Geometry check sheet. Reference: drawing and pictorial views, mm from the part's lowest x, y, z. Give positions to 0.01 mm unless a question says otherwise; leave off trailing zeros. Loops run counter-clockwise (first coordinate to the right, second up) from the corner with the lowest first, then second, coordinate; pieces in that order, holes last. Notation, with made-up numbers: M -12.75,-14.75 L 24.25,-14.75 A15 ccw 24.25,6.25 Z; hole C 5,33.5 d9. An arc over 180 degrees is marked long. Use CSV: the item, a comma, the result in double quotes.
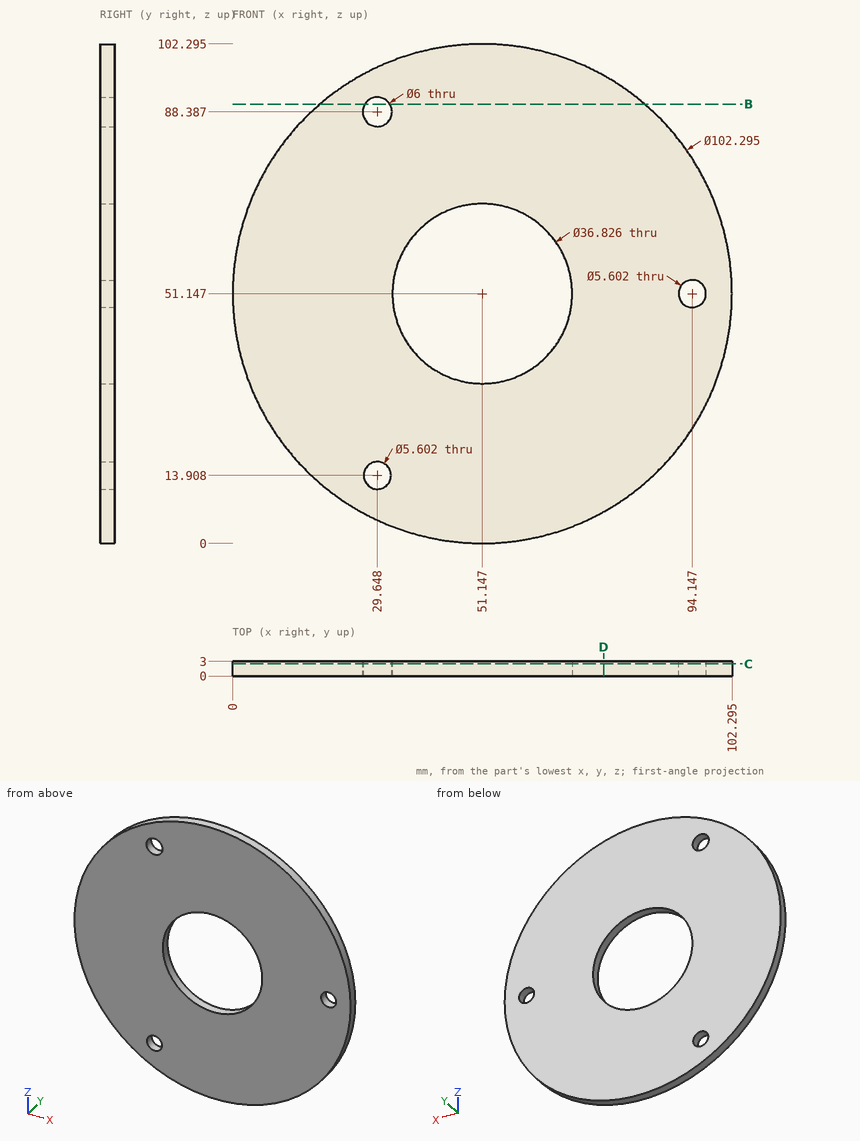
(1) Depth check by flat-ended pin: pin 1 Ø1 at (x, y) = (60, 1.5) entering from -Z; pin 2 Ø1.5 at (x, y) = (30, 1) entering from +Z. Enter the tip coordinate at first touch or a pass-through.
Calculated:
pin 1,"stops at z = 0.69"
pin 2,"stops at z = 98.05"
(2) Section check B-B on z = 90. Record the cut outline in (x, y).
Calculated:
outline,"M 17.88,0 L 27.12,0 L 27.12,3 L 17.88,3 Z; M 32.18,0 L 84.41,0 L 84.41,3 L 32.18,3 Z"
(3) Section check C-C on y = 2.5. Record the cut outline in (x, z) (1 decimal), plus the area to 3 significant figures.
Calculated:
outline,"C 51.1,51.1 d102.3; hole C 29.6,88.4 d6; hole C 29.6,13.9 d5.6; hole C 51.1,51.1 d36.8; hole C 94.1,51.1 d5.6"
area,"7,080 mm²"
(4) Scan lines: L1, parallel to Z at x = 37.5, y = 1.95 (1 decimal); L2, parallel to Z at x = 45, y = 1.7 (1 decimal); L3, parallel to X at y = 1.8, z = 87 (1 decimal). Record each from-to range of solid material in increasing order. Write a range as from..to.
Calculated:
L1,"z = 1.9..38.8, 63.5..100.4"
L2,"z = 0.4..33.8, 68.5..101.9"
L3,"x = 14.7..27, 32.3..87.6"
(5) Section check D-D on x = 76. Record the cut outline in (y, z), plus the area to 3 significant figures.
Calculated:
outline,"M 0,6.44 L 3,6.44 L 3,95.85 L 0,95.85 Z"
area,"268 mm²"
